```python
from build123d import *

# Parameters (mm, degrees)
SKETCH1_R                                      = 17.78
BOSS_EXTRUDE1_DEPTH                            = 6.35
CBORE_FOR_6_SOCKET_HEAD_CAP_SCREW1_D           = 3.6576
CBORE_FOR_6_SOCKET_HEAD_CAP_SCREW1_CBORE_D     = 7.14502
CBORE_FOR_6_SOCKET_HEAD_CAP_SCREW1_CBORE_DEPTH = 3.5052
CIRPATTERN1_COUNT                              = 3
CIRPATTERN3_COUNT                              = 3
CBORE_FOR_6_SOCKET_HEAD_CAP_SCREW2_D           = 3.6576
CBORE_FOR_6_SOCKET_HEAD_CAP_SCREW2_CBORE_D     = 7.14502
CBORE_FOR_6_SOCKET_HEAD_CAP_SCREW2_CBORE_DEPTH = 3.5052
CIRPATTERN4_COUNT                              = 3
SKETCH19_R                                     = 1.27
CUT_EXTRUDE1_DEPTH                             = 26.934134043
CIRPATTERN5_COUNT                              = 3


with BuildPart() as part:
    # Sketch1 → Boss-Extrude1 (new body)
    with BuildSketch(Plane(origin=(0, 0, 0), x_dir=(1, 0, 0), z_dir=(0, 1, 0))):
        with Locations(Location((0, 0, 0), (0, 0, 270))):
            Circle(SKETCH1_R)
    extrude(amount=BOSS_EXTRUDE1_DEPTH)

    # CBORE for #6 Socket Head Cap Screw1 (through all)
    with Locations(Plane(origin=(0, 6.35, 0), x_dir=(1, 0, 0), z_dir=(0, 1, 0))):
        with Locations((7.755232511, -9.242326206)):
            cbore_for_6_socket_head_cap_screw1 = CounterBoreHole(CBORE_FOR_6_SOCKET_HEAD_CAP_SCREW1_D / 2, CBORE_FOR_6_SOCKET_HEAD_CAP_SCREW1_CBORE_D / 2, CBORE_FOR_6_SOCKET_HEAD_CAP_SCREW1_CBORE_DEPTH)

    # CirPattern1: CBORE for #6 Socket Head Cap Screw1 ×3 about axis
    cirpattern1_axis = Axis((0, 0, 0), (0, 1, 0))
    for i in range(1, CIRPATTERN1_COUNT):
        add(cbore_for_6_socket_head_cap_screw1.rotate(cirpattern1_axis, i * 360 / CIRPATTERN1_COUNT), mode=Mode.SUBTRACT)

    # Sketch15 → Tap Drill for #2-56 Tap1 (revolve, cut)
    with BuildSketch(Plane(origin=(-8.835910942, 3.105629072, 15.4290336), x_dir=(0.8677746681735184, 0, 0.49695787072581915), z_dir=(0, 1, 0))):
        Polygon((0, 0), (0, 7.095959572), (0.889, 6.35), (0.889, 0), align=None)
    tap_drill_for_2_56_tap1 = revolve(axis=Axis((-11.991593421, 3.105629072, 20.939402743), (0.49695787072581915, 0, -0.8677746681735184)), mode=Mode.SUBTRACT)

    # CirPattern3: Tap Drill for #2-56 Tap1 ×3 about axis
    cirpattern3_axis = Axis((0, 6.35, 0), (0, -1, 0))
    for i in range(1, CIRPATTERN3_COUNT):
        add(tap_drill_for_2_56_tap1.rotate(cirpattern3_axis, i * 360 / CIRPATTERN3_COUNT), mode=Mode.SUBTRACT)

    # CBORE for #6 Socket Head Cap Screw2 (through all)
    with Locations(Plane(origin=(10.448596497, 0, -6.0325), x_dir=(0, 0, -1), z_dir=(0, -1, 0))):
        with Locations((0, 0)):
            cbore_for_6_socket_head_cap_screw2 = CounterBoreHole(CBORE_FOR_6_SOCKET_HEAD_CAP_SCREW2_D / 2, CBORE_FOR_6_SOCKET_HEAD_CAP_SCREW2_CBORE_D / 2, CBORE_FOR_6_SOCKET_HEAD_CAP_SCREW2_CBORE_DEPTH)

    # CirPattern4: CBORE for #6 Socket Head Cap Screw2 ×3 about axis
    cirpattern4_axis = Axis((0, 0, 0), (0, 1, 0))
    for i in range(1, CIRPATTERN4_COUNT):
        add(cbore_for_6_socket_head_cap_screw2.rotate(cirpattern4_axis, i * 360 / CIRPATTERN4_COUNT), mode=Mode.SUBTRACT)

    # Sketch19 → Cut-Extrude1 (cut, through all)
    with BuildSketch(Plane(origin=(0, 6.35, 0), x_dir=(1, 0, 0), z_dir=(0, 1, 0))):
        with Locations(Location((11.33739147, -4.126473029, 0), (0, 0, 270))):
            Circle(SKETCH19_R)
    cut_extrude1 = extrude(amount=-CUT_EXTRUDE1_DEPTH, mode=Mode.SUBTRACT)

    # CirPattern5: Cut-Extrude1 ×3 about axis
    cirpattern5_axis = Axis((0, 0, 0), (0, 1, 0))
    for i in range(1, CIRPATTERN5_COUNT):
        add(cut_extrude1.rotate(cirpattern5_axis, i * 360 / CIRPATTERN5_COUNT), mode=Mode.SUBTRACT)


solid = part.part
```
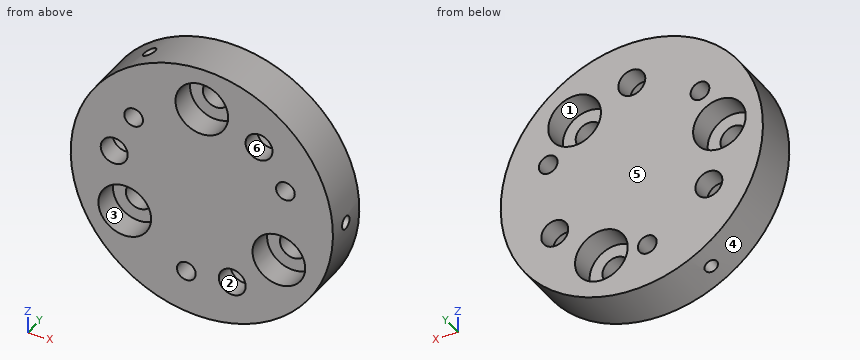
The model under review builds one solid part; all positions refer to its coordinate system, in mm. Face numbers are marked on the shaded views. A direction names the side the tool comes from. Give positions to 0.01 mm unless a question says otherwise; leave off trailing zeros. Write each loop counter-clockwise with the first axis right and the second up, starting at its lowest first coordinate (ties: lowest second). Pieces come first, ordered by that corner, then holes. Notation, with made-up numbers: (41.25, -17.5) -> (92.25, -17.5) arc R28 cw to (92.25, 19.5) -> close; hole circle Ø2 at (-21, 61.5). An arc over 180 degrees is marked (long way). Answer in a Markdown table with one row per item.
1) Clearance check with flat-ended pins moving along their axes: P1, Ø2, axis at x = 11.34, z = 4.13, coming from the -Y side; P2, Ø4.5, axis at x = 10.45, z = -6.03, coming from the +Y side; P3, Ø1.5, axis at y = 3.5, z = -7, coming from the +X side; P4, Ø6, axis at x = 0, z = 12.065, coming from the -Y side. State where each tip first meets the part, or that it passes through.
Worked answers:
| item | result |
|---|---|
| P1 | through |
| P2 | y = 6.35 |
| P3 | x = 16.65 |
| P4 | y = 3.51 |
2) Tool access review of the marked faces 1, 2 and 3: name each direction out of +Z, -Z, +X, -X, +Y, -Y from which nothing blocks a thin tool from reaching the whole face with its end or side.
Worked answers:
| item | result |
|---|---|
| face 1 | +Y |
| face 2 | +Y, -Y |
| face 3 | -Y |
3) Add section B-B on y = 5.5. Count the separate pieces of the cut face and the enclosed holes in it, plus the area to 3 significant figures.
Worked answers:
| item | result |
|---|---|
| separate pieces | 1 |
| enclosed holes | 9 |
| area | 826 mm² |
4) Add section A-A on x = 0. State the section outline as (y, z) points.
Worked answers:
| item | result |
|---|---|
| outline | (0, -17.78) -> (6.35, -17.78) -> (6.35, 10.24) -> (3.51, 10.24) -> (3.51, 8.49) -> (0, 8.49) -> close; (0, 15.64) -> (3.51, 15.64) -> (3.51, 13.89) -> (6.35, 13.89) -> (6.35, 17.78) -> (0, 17.78) -> close |
5) Mouldability with a two-part tool opening along Z and no side actions: class the marked faces 4, 5 and 6 as +Z half, -Z half, draft (parallel to the pull), parting line (faces both ways), or undercut.
Worked answers:
| item | result |
|---|---|
| face 4 | parting line |
| face 5 | draft |
| face 6 | undercut |
6) For L1, parallel to X at y = 2, z = -7; L2, parallel to X at y = 3.25, z = -4; L3, parallel to Z at x = -2, y = 1, list the stretches that pass through material, from the lowest coordinate up. Write a range as [from, to].
Worked answers:
| item | result |
|---|---|
| L1 | [-16.34, -13.89], [-7.01, 7.01], [13.89, 16.34] |
| L2 | [-17.32, -13.39], [-7.51, 7.51], [13.39, 17.32] |
| L3 | [-17.67, -13.15], [-10.62, 9.1], [15.03, 17.67] |
